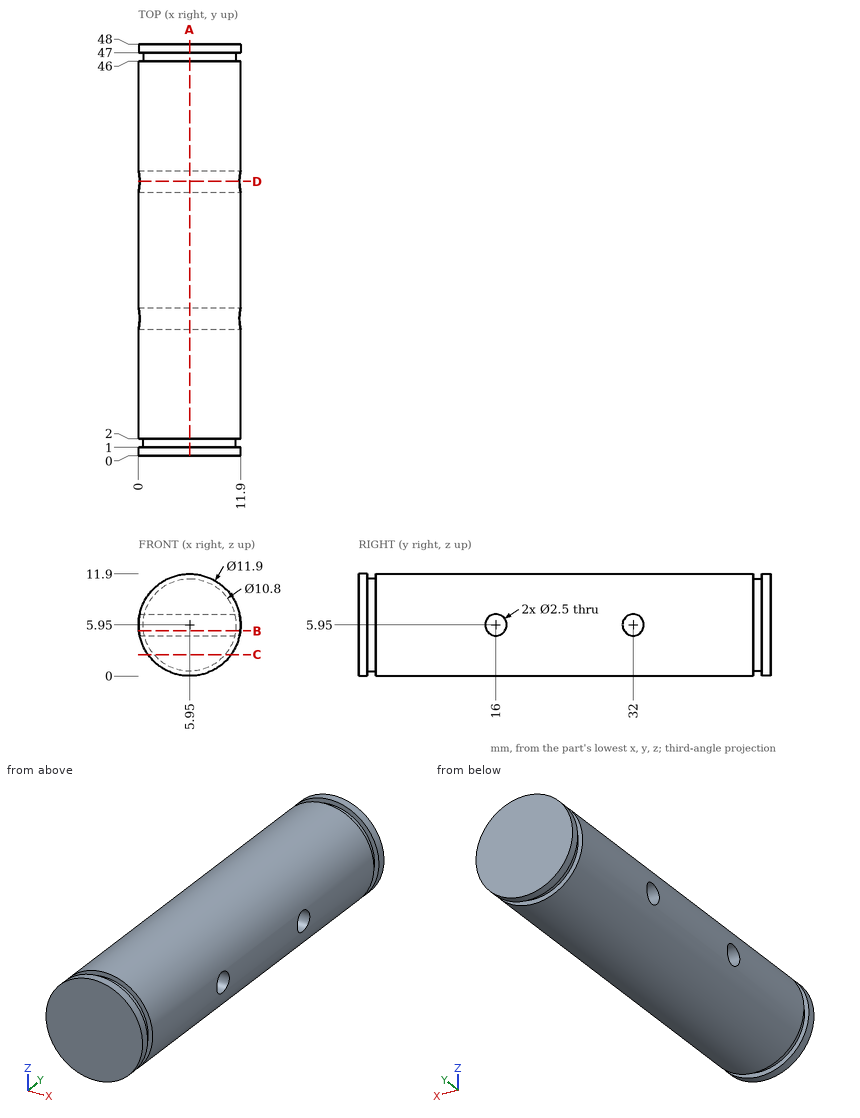
Source: three-view drawing plus pictorial views. Frame: mm from the lowest corner of the part. Give positions to 0.01 mm unless a question says otherwise; leave off trailing zeros. Write each loop counter-clockwise with the first axis right and the second up, starting at its lowest first coordinate (ties: lowest second). Pieces come first, ordered by that corner, then holes.
(1) Cut plane D-D, the plane y = 32. Return loops of the section in (x, z), then the cut area to 3 significant figures.
(2) Cut plane C-C, the plane z = 2.5. Return loops of the section in (x, y).
(3) First-contact query: P1, Ø2, axis at y = 16, z = 5.95, coming from the +X side; P2, Ø1, axis at x = 3.5, z = 8, coming from the -Y side; P3, Ø1.5, axis at y = 30, z = 4, coming from the +X side; P4, Ø5, axis at y = 28, z = 10.5, coming from the -X side. Flat tips, straight axial feed; report the tip coordinate or a pass-through.
(4) Cut plane B-B, the plane z = 5.25. Return loops of the section in (x, y).
(5) Cut plane A-A, the plane x = 5.95. Return loops of the section in (y, z), then the cut area to 3 significant figures.
(6) Ray query, line 1 (Y direction, x = 4.5, z = 5.95); line 2 (Y direction, x = 1, z = 3.5); line 3 (Z direction, x = 6.25, y = 16). Return the intervals inside material, ascending.
Values follow:
1. outline: (0.13, 4.7) arc R5.95 ccw to (11.77, 4.7) - close; (0.13, 7.2) - (11.77, 7.2) arc R5.95 ccw to start
1. area: 81.7 mm2
2. outline: (1.1, 0) - (10.8, 0) - (10.8, 1) - (10.1, 1) - (10.1, 2) - (10.8, 2) - (10.8, 46) - (10.1, 46) - (10.1, 47) - (10.8, 47) - (10.8, 48) - (1.1, 48) - (1.1, 47) - (1.8, 47) - (1.8, 46) - (1.1, 46) - (1.1, 2) - (1.8, 2) - (1.8, 1) - (1.1, 1) - close
3. P1: passes through
3. P2: stops at y = 0
3. P3: stops at x = 11.78
3. P4: stops at x = 0.36
4. outline: (0.04, 0) - (11.86, 0) - (11.86, 1) - (11.3, 1) - (11.3, 2) - (11.86, 2) - (11.86, 14.96) - (0.04, 14.96) - (0.04, 2) - (0.6, 2) - (0.6, 1) - (0.04, 1) - close; (0.04, 17.04) - (11.86, 17.04) - (11.86, 30.96) - (0.04, 30.96) - close; (0.04, 33.04) - (11.86, 33.04) - (11.86, 46) - (11.3, 46) - (11.3, 47) - (11.86, 47) - (11.86, 48) - (0.04, 48) - (0.04, 47) - (0.6, 47) - (0.6, 46) - (0.04, 46) - close
5. outline: (0, 0) - (1, 0) - (1, 0.55) - (2, 0.55) - (2, 0) - (46, 0) - (46, 0.55) - (47, 0.55) - (47, 0) - (48, 0) - (48, 11.9) - (47, 11.9) - (47, 11.35) - (46, 11.35) - (46, 11.9) - (2, 11.9) - (2, 11.35) - (1, 11.35) - (1, 11.9) - (0, 11.9) - close; hole circle Ø2.5 at (16, 5.95); hole circle Ø2.5 at (32, 5.95)
5. area: 559 mm2
6. line 1: y = 0 to 14.75, 17.25 to 30.75, 33.25 to 48
6. line 2: y = 0 to 1, 2 to 46, 47 to 48
6. line 3: z = 0.01 to 4.7, 7.2 to 11.89
